Geometry check sheet. Reference: the model listing, model coordinates, mm. A direction names the side the tool comes from. Round coordinates to 2 decimals unless told otherwise and drop trailing zeros. Loops run counter-clockwise (first coordinate to the right, second up) from the corner with the lowest first, then second, coordinate; pieces in that order, holes last. Notation, with made-up numbers: (10, 73.25) -> (53, 73.25) arc R27 ccw to (53, 92.25) -> close; hole circle Ø3 at (-25.5, 14). An arc over 180 degrees is marked (long way). Use a Markdown table: item, result. Add a question column.
Q1. Gauge pin test, flat ends, axial feed: P1, Ø0.8, axis at x = -82, y = 1, coming from the -Z side; P2, Ø1.8, axis at x = 27, y = 4.5, coming from the -Z side; P3, Ø6, axis at x = -3, z = -22, coming from the -Y side. Record the tip position at first contact, or that the pin passes through.
Q2. Sectioned sample at A-A, the plane y = 4.75. Enter the section's corners in (x, z), then the cut area to 3 significant figures.
Q3. Release check for a two-part mould opening along Y. For faces 5 (the face through (-47.106, 5, -62)), 6 (the face through (-65.106, 2, -62)), 7 (the face through (51, 0, -62)) record: released by +Y, released by -Y, zero draft, split by the parting line, or undercut.
Q4. Set-up check for faces 1 (the face through (-69, 3, -53.347)), 2 (the face through (-8, 4, 42.653)), 3 (the face through (26.911, 2, -62)), 4 (the face through (31, 3, -62)): record each of +Z, -Z, +X, -X, +Y, -Y from which the full face is reachable in a straight line by a thin tool's end or side.
Q5. Material ranges on L1, parallel to Z at x = 52, y = 2.25; L2, parallel to X at y = 5.75, z = 33.5; L3, parallel to X at y = 0.5, z = 18, recorded low to high.
```python
from build123d import *

# Parameters (mm, degrees)
F1_DEPTH  = 8.6
F2_T      = -2.1
F3_DEPTH  = 25
F4_W      = 2.5
F4_H      = 108.4
F5_DEPTH  = 3
F5_TAPER  = -2
F6_W      = 3
F6_H      = 17
F7_DEPTH  = 3.5
F8_W      = 6
F8_H      = 17
F9_DEPTH  = 3
F10_W     = 2.4673982024
F10_H     = 22.8933023606
F11_DEPTH = 4


with BuildPart() as f1:
    # F0 (on Front) → F1 (new body)
    with BuildSketch(Plane.XZ):
        Polygon((0, 42.6528545822), (-85.1061937809, 42.6528545822), (-85.1061937809, -70.3471454178), (-68.1061937809, -70.3471454178), (-65.1061937809, -70.3471454178), (-44.1061937809, -70.3471454178), (-41.1061937809, -70.3471454178), (0, -70.3471454178), align=None)
        Polygon((67.8938062191, 42.6528545822), (0, 42.6528545822), (0, -70.3471454178), (23.8938062191, -70.3471454178), (26.8938062191, -70.3471454178), (47.8938062191, -70.3471454178), (50.8938062191, -70.3471454178), (67.8938062191, -70.3471454178), align=None)
    extrude(amount=-F1_DEPTH)

    # F2
    f2_openings = [f1.faces().sort_by_distance(p)[0] for p in [
        (-8.606194, 0, -13.847145),
    ]]
    offset(amount=F2_T, openings=f2_openings)

    # F3 (cut): a face of the model
    f3_faces = [f1.faces().sort_by_distance(p)[0] for p in [
        (-8.6061937809, 3.25, -68.2471454178),
    ]]
    extrude(f3_faces, amount=-F3_DEPTH, mode=Mode.SUBTRACT)

    # F4 (on face) → F5 (join)
    with BuildSketch(Plane.XZ):
        Polygon((-80.5061937809, 40.5528545822), (-80.5061937809, 38.0528545822), (63.2938062191, 38.0528545822), (65.7938062191, 38.0528545822), (65.7938062191, 40.5528545822), align=None)
        Polygon((-83.0061937809, 40.5528545822), (-83.0061937809, -70.3471454178), (-80.5061937809, -70.3471454178), (-80.5061937809, 38.0528545822), (-80.5061937809, 40.5528545822), align=None)
        with Locations((64.5438062191, -16.1471454178)):
            Rectangle(F4_W, F4_H)
    extrude(amount=-F5_DEPTH, taper=F5_TAPER)

    # F6 (on face) → F7 (join)
    with BuildSketch(Plane.XZ.offset(-6.5)):
        with Locations((-69.6061937809, -61.8471454178)):
            Rectangle(F6_W, F6_H)
        with Locations((-45.6061937809, -61.8471454178)):
            Rectangle(F6_W, F6_H)
        with Locations((28.3938062191, -61.8471454178)):
            Rectangle(F6_W, F6_H)
        with Locations((52.3938062191, -61.8471454178)):
            Rectangle(F6_W, F6_H)
    extrude(amount=F7_DEPTH)

    # F8 (on face) → F9 (join)
    with BuildSketch(Plane.XZ.offset(-3)):
        with Locations((-68.1061937809, -61.8471454178)):
            Rectangle(F8_W, F8_H)
        with Locations((-47.0006712973, -61.8471454178)):
            Rectangle(F8_W, F8_H)
        with Locations((29.9112996757, -61.8471454178)):
            Rectangle(F8_W, F8_H)
        with Locations((50.9397262037, -61.8471454178)):
            Rectangle(F8_W, F8_H)
    extrude(amount=F9_DEPTH)

    # F10 (on face) → F11 (cut)
    with BuildSketch(Plane.XZ):
        with Locations((-81.7398928821, -58.9004942375)):
            Rectangle(F10_W, F10_H)
        Polygon((-82.9735919833, -73.1144845486), (-78.0577212572, -73.1144845486), (-78.0577212572, -47.4538430572), (-80.5061937809, -47.4538430572), (-80.5061937809, -70.3471454178), (-82.9735919833, -70.3471454178), align=None)
    extrude(amount=-F11_DEPTH, mode=Mode.SUBTRACT)


solid = f1.part
```
Values:
| question | item | result |
|---|---|---|
| 1 | P1 | z = -47.45 |
| 1 | P2 | z = -70.35 |
| 1 | P3 | y = 6.5 |
| 2 | outline | (-85.11, -70.35) -> (-83.01, -70.35) -> (-83.01, 40.55) -> (65.79, 40.55) -> (65.79, -70.35) -> (67.89, -70.35) -> (67.89, 42.65) -> (-85.11, 42.65) -> close; (-71.11, -70.35) -> (-68.11, -70.35) -> (-68.11, -53.35) -> (-71.11, -53.35) -> close; (-47.11, -70.35) -> (-44.11, -70.35) -> (-44.11, -53.35) -> (-47.11, -53.35) -> close; (26.89, -70.35) -> (29.89, -70.35) -> (29.89, -53.35) -> (26.89, -53.35) -> close; (50.89, -70.35) -> (53.89, -70.35) -> (53.89, -53.35) -> (50.89, -53.35) -> close |
| 2 | area | 991 mm^2 |
| 3 | face 5 | undercut |
| 3 | face 6 | zero draft |
| 3 | face 7 | released by -Y |
| 4 | face 1 | -Y |
| 4 | face 2 | +Z, +X, -X, +Y, -Y |
| 4 | face 3 | -Z, -Y |
| 4 | face 4 | -Z |
| 5 | L1 | -70.35 to -53.35, 37.97 to 42.65 |
| 5 | L2 | -85.11 to -83.01, 65.79 to 67.89 |
| 5 | L3 | -85.11 to -80.49, 63.28 to 67.89 |
